from build123d import *

# Parameters (mm, degrees)
SKETCH1_R           = 2
BOSS_EXTRUDE1_DEPTH = 4


with BuildPart() as part:
    # Sketch1 → Boss-Extrude1 (new body)
    with BuildSketch(Plane.XZ):
        with BuildLine():
            Line((-72, -4), (72, -4))
            ThreePointArc((72, -4), (76, 0), (72, 4))
            Line((72, 4), (-72, 4))
            ThreePointArc((-72, 4), (-76, 0), (-72, -4))
        make_face()
        with Locations(Location((-72, 0, 0), (0, 0, 90))):
            Circle(SKETCH1_R, mode=Mode.SUBTRACT)
        with Locations(Location((-64, 0, 0), (0, 0, 90))):
            Circle(SKETCH1_R, mode=Mode.SUBTRACT)
        with Locations(Location((-56, 0, 0), (0, 0, 90))):
            Circle(SKETCH1_R, mode=Mode.SUBTRACT)
        with Locations(Location((-48, 0, 0), (0, 0, 90))):
            Circle(SKETCH1_R, mode=Mode.SUBTRACT)
        with Locations(Location((-40, 0, 0), (0, 0, 90))):
            Circle(SKETCH1_R, mode=Mode.SUBTRACT)
        with Locations(Location((-32, 0, 0), (0, 0, 90))):
            Circle(SKETCH1_R, mode=Mode.SUBTRACT)
        with Locations(Location((-24, 0, 0), (0, 0, 90))):
            Circle(SKETCH1_R, mode=Mode.SUBTRACT)
        with Locations(Location((-16, 0, 0), (0, 0, 90))):
            Circle(SKETCH1_R, mode=Mode.SUBTRACT)
        with Locations(Location((-8, 0, 0), (0, 0, 90))):
            Circle(SKETCH1_R, mode=Mode.SUBTRACT)
        with Locations(Location((0, 0, 0), (0, 0, 90))):
            Circle(SKETCH1_R, mode=Mode.SUBTRACT)
        with Locations(Location((8, 0, 0), (0, 0, 90))):
            Circle(SKETCH1_R, mode=Mode.SUBTRACT)
        with Locations(Location((16, 0, 0), (0, 0, 90))):
            Circle(SKETCH1_R, mode=Mode.SUBTRACT)
        with Locations(Location((24, 0, 0), (0, 0, 90))):
            Circle(SKETCH1_R, mode=Mode.SUBTRACT)
        with Locations(Location((32, 0, 0), (0, 0, 90))):
            Circle(SKETCH1_R, mode=Mode.SUBTRACT)
        with Locations(Location((40, 0, 0), (0, 0, 90))):
            Circle(SKETCH1_R, mode=Mode.SUBTRACT)
        with Locations(Location((48, 0, 0), (0, 0, 90))):
            Circle(SKETCH1_R, mode=Mode.SUBTRACT)
        with Locations(Location((56, 0, 0), (0, 0, 90))):
            Circle(SKETCH1_R, mode=Mode.SUBTRACT)
        with Locations(Location((64, 0, 0), (0, 0, 90))):
            Circle(SKETCH1_R, mode=Mode.SUBTRACT)
        with Locations(Location((72, 0, 0), (0, 0, 90))):
            Circle(SKETCH1_R, mode=Mode.SUBTRACT)
    extrude(amount=-BOSS_EXTRUDE1_DEPTH)


solid = part.part
Could you check a few things on this model? Use its own coordinates, in mm. Round coordinates to 2 decimals unless told otherwise and drop trailing zeros. Order: outer loops, then holes, each group sorted by start corner. A loop starts at its lowest first (then second) coordinate and runs counter-clockwise, first axis right, second up.
Q1. Please list where these lines run through material, in increasing order: probe 1 along Z at (x, y) = (-24, 1.4); probe 2 along X at (y, z) = (1.2, 3); probe 3 along X at (y, z) = (3.7, -2.75).
Geometry says:
probe 1: z = -4 to -2, 2 to 4
probe 2: x = -74.65 to 74.65
probe 3: x = -74.9 to 74.9
Q2. Thinking about a two-plate mould opening in X: for faces 1 (the face through (-58, 2, 0)), 2 (the face through (-76, 2, 0)), 3 (the face through (76, 2, 0)), 4 (the face through (-1, 2, -4)), which applies, released by +X, released by -X, zero draft, split by the parting line, or undercut?
Geometry says:
face 1: undercut
face 2: released by -X
face 3: released by +X
face 4: zero draft
Q3. Imagine slicing it at B-B, the plane y = 3.4. State how many separate pieces and enclosed holes the cut face has, then the cut area to 3 significant figures.
Geometry says:
separate pieces: 1
enclosed holes: 19
area: 964 mm2
Q4. I'm going to push flat-ended pins straight in: P1, Ø1.5, axis at x = 27.5, z = 0, coming from the -Y side; P2, Ø1, axis at y = 1.5, z = -1.5, coming from the -X side; P3, Ø1, axis at y = 1.5, z = -2.5, coming from the +X side. Where does each tip first touch, or does it pass through?
Geometry says:
P1: stops at y = 0
P2: stops at x = -75.87
P3: stops at x = 75.46
Q5. Imagine slicing it at A-A, the plane x = 16. List the corners of the cut face in (y, z) for me, then the cut area to 3 significant figures.
Geometry says:
outline: (0, -4) - (4, -4) - (4, -2) - (0, -2) - close; (0, 2) - (4, 2) - (4, 4) - (0, 4) - close
area: 16.0 mm2
